```python
from build123d import *

# Parameters (mm, degrees)
ESQUISSE1_R                  = 25
BOSS_EXTRU_1_DEPTH           = 8
ESQUISSE2_R                  = 14
BOSS_EXTRU_2_DEPTH           = 40
ENL_V_MAT_EXTRU_1_DEPTH      = 60.615434243
ENL_V_MAT_EXTRU_1_DEPTH_BACK = 60.615434243
ESQUISSE3_R                  = 10
ENL_V_MAT_EXTRU_2_DEPTH      = 54.38539126
ENL_V_MAT_EXTRU_2_DEPTH_BACK = 54.38539126
ESQUISSE4_R                  = 2.75


with BuildPart() as part:
    # Esquisse1 → Boss.-Extru.1 (new body)
    with BuildSketch(Plane(origin=(0, 0, 0), x_dir=(1, 0, 0), z_dir=(0, 1, 0))):
        with Locations(Location((0, 0, 0), (0, 0, 270))):
            Circle(ESQUISSE1_R)
    extrude(amount=BOSS_EXTRU_1_DEPTH)

    # Esquisse2 → Boss.-Extru.2 (add)
    with BuildSketch(Plane(origin=(0, 8, 0), x_dir=(1, 0, 0), z_dir=(0, 1, 0))):
        with Locations(Location((0, 0, 0), (0, 0, 270))):
            Circle(ESQUISSE2_R)
    extrude(amount=BOSS_EXTRU_2_DEPTH)

    # Esquisse3 → Enlèv. mat.-Extru.1 (cut, two sides: drawn at the far end of the back side and taken through both)
    with BuildSketch(Plane(origin=(0, 48, 0), x_dir=(1, 0, 0), z_dir=(0, 1, 0)).offset(-ENL_V_MAT_EXTRU_1_DEPTH_BACK)):
        with Locations(Location((0, 0, 0), (0, 0, 270))):
            Circle(ESQUISSE3_R)
    extrude(amount=ENL_V_MAT_EXTRU_1_DEPTH + ENL_V_MAT_EXTRU_1_DEPTH_BACK, mode=Mode.SUBTRACT)

    # Esquisse4 → Enlèv. mat.-Extru.2 (cut, two sides: drawn at the far end of the back side and taken through both)
    with BuildSketch(Plane(origin=(0, 8, 0), x_dir=(1, 0, 0), z_dir=(0, 1, 0)).offset(-ENL_V_MAT_EXTRU_2_DEPTH_BACK)):
        with Locations(Location((0, 20, 0), (0, 0, 270))):
            Circle(ESQUISSE4_R)
        with Locations(Location((20, 0, 0), (0, 0, 270))):
            Circle(ESQUISSE4_R)
        with Locations(Location((0, -20, 0), (0, 0, 270))):
            Circle(ESQUISSE4_R)
        with Locations(Location((-20, 0, 0), (0, 0, 270))):
            Circle(ESQUISSE4_R)
    extrude(amount=ENL_V_MAT_EXTRU_2_DEPTH + ENL_V_MAT_EXTRU_2_DEPTH_BACK, mode=Mode.SUBTRACT)


solid = part.part
```
Read the model definition and answer for the solid it produces. Units are mm, in the model's axes. Coordinates: 2 decimals unless noted, no trailing zeros. Write each loop counter-clockwise with the first axis right and the second up, starting at its lowest first coordinate (ties: lowest second). Pieces come first, ordered by that corner, then holes. Notation, with made-up numbers: (44, 52.5) -> (61, 52.5) arc R32 ccw to (61, 81.5) -> close; hole circle Ø4 at (80.25, 39). An arc over 180 degrees is marked (long way). Answer as a JSON object with one key per item and string values.
Q1. Determine the mould class of faces 1 (the flat face through (-11, 8, 11)), 2 (the cylindrical face through (-13.67, 27.72, -3.03)), 3 (the cylindrical face through (22.727, 3.944, -0.358)) for opening direction X: pulls with the +X half, pulls with the -X half, needs draft (parallel to the pull), parting line crosses it, or undercut.
The answers:
{"face 1": "needs draft", "face 2": "parting line crosses it", "face 3": "undercut"}
Q2. Consider line 1 (X direction, y = 4.5, z = 0); line 2 (X direction, y = 18.5, z = -0.5); line 3 (Y direction, x = -17, z = -10). Determine where each line is inside the solid, lowest interval first. Write a range as [from, to].
The answers:
{"line 1": "x = [-25, -22.75], [-17.25, -10], [10, 17.25], [22.75, 25]", "line 2": "x = [-13.99, -9.99], [9.99, 13.99]", "line 3": "y = [0, 8]"}
Q3. The part is cut by section C-C on x = 20. Give the vertices of the cut face in (y, z), then the cut area to 3 significant figures.
The answers:
{"outline": "(0, -15) -> (8, -15) -> (8, -2.75) -> (0, -2.75) -> close; (0, 2.75) -> (8, 2.75) -> (8, 15) -> (0, 15) -> close", "area": "196 mm2"}
Q4. Flat-ended cylindrical pins translate along their axes: pin 1 Ø2 at (y, z) = (18, -8) entering from -X; pin 2 Ø3 at (y, z) = (22.5, 11) entering from -X; pin 3 Ø8 at (x, y) = (15, 40) entering from +Z. Find the tip coordinate at first contact, or state that the pin passes through.
The answers:
{"pin 1": "stops at x = -12.12", "pin 2": "stops at x = -10.28", "pin 3": "stops at z = 8.66"}
Q5. The part is cut by section D-D on z = 0. Give the vertices of the cut face in (x, y).
The answers:
{"outline": "(-25, 0) -> (-22.75, 0) -> (-22.75, 8) -> (-25, 8) -> close; (-17.25, 0) -> (-10, 0) -> (-10, 48) -> (-14, 48) -> (-14, 8) -> (-17.25, 8) -> close; (10, 0) -> (17.25, 0) -> (17.25, 8) -> (14, 8) -> (14, 48) -> (10, 48) -> close; (22.75, 0) -> (25, 0) -> (25, 8) -> (22.75, 8) -> close"}
Q6. The part is cut by section A-A on x = 0. Give the vertices of the cut face in (y, z).
The answers:
{"outline": "(0, -25) -> (8, -25) -> (8, -22.75) -> (0, -22.75) -> close; (0, -17.25) -> (8, -17.25) -> (8, -14) -> (48, -14) -> (48, -10) -> (0, -10) -> close; (0, 10) -> (48, 10) -> (48, 14) -> (8, 14) -> (8, 17.25) -> (0, 17.25) -> close; (0, 22.75) -> (8, 22.75) -> (8, 25) -> (0, 25) -> close"}
Q7. The part is cut by section B-B on z = 20. Give the vertices of the cut face in (x, y), then the cut area to 3 significant figures.
The answers:
{"outline": "(-15, 0) -> (-2.75, 0) -> (-2.75, 8) -> (-15, 8) -> close; (2.75, 0) -> (15, 0) -> (15, 8) -> (2.75, 8) -> close", "area": "196 mm2"}
